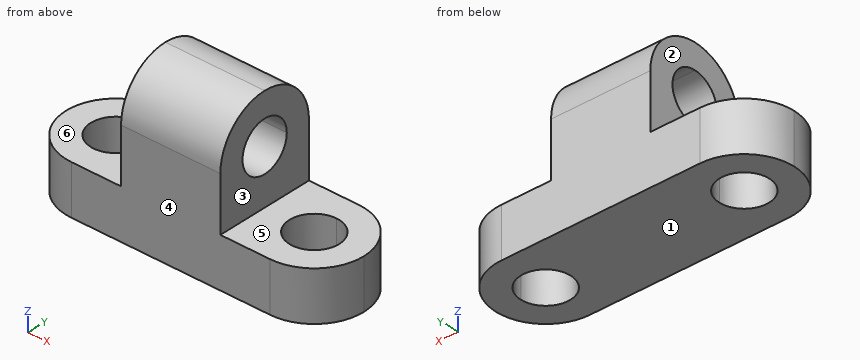
from build123d import *

# Parameters (mm, degrees)
F1_DEPTH  = 25.4
F3_DEPTH  = 25.4
F5_DEPTH  = 25.4
F7_DEPTH  = 25.4
F9_DEPTH  = 25.4
F11_DEPTH = 25.4
F13_DEPTH = 25.4
F15_DEPTH = 25.4


with BuildPart() as f1:
    # F0 (on Front) → F1 (new body)
    with BuildSketch(Plane.XZ):
        Polygon((-49.976994, -0.463082), (-49.976994, -13.163082), (26.223006, -13.163082), (26.223006, -0.463082), (0.823006, -0.463082), (0.823006, 26.227836), (-24.576994, 26.227836), (-24.576994, -0.463082), align=None)
    extrude(amount=F1_DEPTH)

    # F2 (on face) → F3 (cut)
    with BuildSketch(Plane.YZ.offset(0.823006)):
        with BuildLine():
            Line((-25.4, 26.227836), (-25.4, 13.527836))
            ThreePointArc((-25.4, 13.527836), (-21.680256, 22.508093), (-12.7, 26.227836))
            Line((-12.7, 26.227836), (-25.4, 26.227836))
        make_face()
        with BuildLine():
            Line((0, 26.227836), (-12.7, 26.227836))
            ThreePointArc((-12.7, 26.227836), (-3.719744, 22.508093), (0, 13.527836))
            Line((0, 13.527836), (0, 26.227836))
        make_face()
    extrude(amount=-F3_DEPTH, mode=Mode.SUBTRACT)

    # F4 (on face) → F5 (cut)
    with BuildSketch(Plane.XY.offset(-0.463082)):
        with BuildLine():
            Line((26.223006, 0), (13.523006, 0))
            ThreePointArc((13.523006, 0), (22.503262, -3.719744), (26.223006, -12.7))
            Line((26.223006, -12.7), (26.223006, 0))
        make_face()
        with BuildLine():
            Line((26.223006, -25.4), (26.223006, -12.7))
            ThreePointArc((26.223006, -12.7), (22.503262, -21.680256), (13.523006, -25.4))
            Line((13.523006, -25.4), (26.223006, -25.4))
        make_face()
    extrude(amount=-F5_DEPTH, mode=Mode.SUBTRACT)

    # F6 (on face) → F7 (cut)
    with BuildSketch(Plane.XY.offset(-0.463082)):
        with BuildLine():
            ThreePointArc((-37.276994, -25.4), (-46.25725, -21.680256), (-49.976994, -12.7))
            Line((-49.976994, -12.7), (-49.976994, -25.4))
            Line((-49.976994, -25.4), (-37.276994, -25.4))
        make_face()
    extrude(amount=-F7_DEPTH, mode=Mode.SUBTRACT)

    # F8 (on face) → F9 (cut)
    with BuildSketch(Plane.XY.offset(-0.463082)):
        with BuildLine():
            ThreePointArc((-37.276994, -25.4), (-46.25725, -21.680256), (-49.976994, -12.7))
            Line((-49.976994, -12.7), (-49.976994, -25.4))
            Line((-49.976994, -25.4), (-37.276994, -25.4))
        make_face()
        with BuildLine():
            ThreePointArc((-49.976994, -12.7), (-46.25725, -3.719744), (-37.276994, 0))
            Line((-37.276994, 0), (-49.976994, 0))
            Line((-49.976994, 0), (-49.976994, -12.7))
        make_face()
    extrude(amount=-F9_DEPTH, mode=Mode.SUBTRACT)

    # F10 (on face) → F11 (cut)
    with BuildSketch(Plane.XY.offset(-0.463082)):
        with BuildLine():
            ThreePointArc((-37.276994, -6.35), (-41.767122, -17.190128), (-30.926994, -12.7))
            ThreePointArc((-30.926994, -12.7), (-32.786866, -8.209872), (-37.276994, -6.35))
        make_face()
    extrude(amount=-F11_DEPTH, mode=Mode.SUBTRACT)

    # F12 (on face) → F13 (cut)
    with BuildSketch(Plane.XY.offset(-0.463082)):
        with BuildLine():
            ThreePointArc((13.523006, -6.35), (9.032878, -17.190128), (19.873006, -12.7))
            ThreePointArc((19.873006, -12.7), (18.013134, -8.209872), (13.523006, -6.35))
        make_face()
    extrude(amount=-F13_DEPTH, mode=Mode.SUBTRACT)

    # F14 (on face) → F15 (cut)
    with BuildSketch(Plane.YZ.offset(0.823006)):
        with BuildLine():
            ThreePointArc((-12.80825, 19.876914), (-17.151691, 8.999598), (-6.35, 13.527836))
            ThreePointArc((-6.35, 13.527836), (-8.248309, 18.056075), (-12.80825, 19.876914))
        make_face()
    extrude(amount=-F15_DEPTH, mode=Mode.SUBTRACT)


solid = f1.part
Could you check a few things on this model? Use its own coordinates, in mm. Face numbers are marked on the shaded views. A direction names the side the tool comes from. Give positions to 0.01 mm unless a question says otherwise; leave off trailing zeros. Order: outer loops, then holes, each group sorted by start corner. A loop starts at its lowest first (then second) coordinate and runs counter-clockwise, first axis right, second up. Notation, with made-up numbers: (5.5, 60) -> (20.5, 60) arc R24 cw to (20.5, 96) -> close; hole circle Ø4 at (-14, 23). An arc over 180 degrees is marked (long way). Answer in a Markdown table with one row per item. Add a question column.
Item 1: For the marked faces 4, 5 and 6, which set-ups out of +Z, -Z, +X, -X, +Y, -Y let a thin tool reach every point of the face, with its end or its side?
Item 2: Imagine slicing it at D-D (z = 4). List the corners of the cut face in (x, y) for me, and give its area (3 significant figures).
Item 3: I'm going to push flat-ended pins straight in: P1, Ø11.5, axis at y = -12.7, z = 13.53, coming from the -X side; P2, Ø4, axis at x = -32, y = -5, coming from the +Z side; P3, Ø12, axis at x = -10, y = -19, coming from the +Z side. Where does each tip first touch, or does it pass through?
Item 4: Imagine slicing it at B-B (x = -16). List the corners of the cut face in (y, z) for me, and give its area (3 significant figures).
Item 5: Please list where these lines run through material, in increasing order: probe 1 along X at (y, z) = (-12.7, -8); probe 2 along X at (y, z) = (-7, -7); probe 3 along Z at (x, y) = (-44.5, -8).
Item 6: Imagine slicing it at A-A (y = -17.5). List the corners of the cut face in (x, z) for me, and give its area (3 significant figures).
Item 7: We'd pull the mould along X, two halves only. Please class the marked faces 1, 2 and 3: pulls with the +X half, pulls with the -X half, needs draft (parallel to the pull), parting line crosses it, or undercut.
Item 8: Imagine slicing it at C-C (x = 10.5). List the corners of the cut face in (y, z) for me, and give its area (3 significant figures).
Result:
| question | item | result |
|---|---|---|
| 1 | face 4 | +Z, -Z, +X, -X, -Y |
| 1 | face 5 | +Z, +X, +Y, -Y |
| 1 | face 6 | +Z, -X, +Y, -Y |
| 2 | outline | (-24.58, -25.4) -> (0.82, -25.4) -> (0.82, 0) -> (-24.58, 0) -> close |
| 2 | area | 645 mm2 |
| 3 | P1 | through |
| 3 | P2 | z = -0.46 |
| 3 | P3 | z = 26.22 |
| 4 | outline | (-25.4, -13.16) -> (0, -13.16) -> (0, 13.53) arc R12.7 ccw to (-12.7, 26.23) arc R12.7 ccw to (-25.4, 13.53) -> close; hole (-12.81, 19.88) arc R6.35 ccw (long way) to (-6.35, 13.53) arc R6.35 ccw to start |
| 4 | area | 805 mm2 |
| 5 | probe 1 | -49.98 to -43.63, -30.93 to 7.17, 19.87 to 26.22 |
| 5 | probe 2 | -48.63 to -40.08, -34.48 to 10.72, 16.32 to 24.87 |
| 5 | probe 3 | -13.16 to -0.46 |
| 6 | outline | (-49.03, -13.16) -> (-41.43, -13.16) -> (-41.43, -0.46) -> (-49.03, -0.46) -> close; (-33.12, -13.16) -> (9.37, -13.16) -> (9.37, -0.46) -> (0.82, -0.46) -> (0.82, 9.37) -> (-24.58, 9.37) -> (-24.58, -0.46) -> (-33.12, -0.46) -> close; (-24.58, 17.69) -> (0.82, 17.69) -> (0.82, 25.29) -> (-24.58, 25.29) -> close; (17.68, -13.16) -> (25.28, -13.16) -> (25.28, -0.46) -> (17.68, -0.46) -> close |
| 6 | area | 1,180 mm2 |
| 7 | face 1 | needs draft |
| 7 | face 2 | pulls with the -X half |
| 7 | face 3 | pulls with the +X half |
| 8 | outline | (-25.4, -13.16) -> (-18.28, -13.16) -> (-18.28, -0.46) -> (-25.4, -0.46) -> close; (-7.12, -13.16) -> (0, -13.16) -> (0, -0.46) -> (-7.12, -0.46) -> close |
| 8 | area | 181 mm2 |
